```python
from build123d import *

# Parameters (mm, degrees)
F1_DEPTH = 3.175
F2_W     = 3.175
F2_H     = 25.4
F3_DEPTH = 7.62
F2_R     = 1.27
F4_DEPTH = 7.62
F5_R     = 2.15265
F6_DEPTH = 25.4


# Not quite as in the source:
# - a length typed as a fraction of an inch, garbled in the dataset ("3 / 203.2 mm" for 3/8 in), is restored


with BuildPart() as f1:
    # F0 (on Top) → F1 (new body)
    with BuildSketch(Plane.XY):
        Polygon((-25.4, -43.9940905122), (25.4, -43.9940905122), (50.8, 0), (101.6, 0), (127, 43.9940905122), (101.6, 87.9881810245), (50.8, 87.9881810245), (25.4, 131.9822715367), (-25.4, 131.9822715367), (-50.8, 87.9881810245), (-101.6, 87.9881810245), (-127, 43.9940905122), (-101.6, 0), (-50.8, 0), align=None)
    extrude(amount=F1_DEPTH)

    # F2 (on face) → F3 (cut)
    with BuildSketch(Plane.XY.offset(3.175)):
        with Locations((-21.59, 69.3940905122)):
            Rectangle(F2_W, F2_H)
        with Locations((21.59, 69.3940905122)):
            Rectangle(F2_W, F2_H)
        with Locations((21.59, 18.5940905122)):
            Rectangle(F2_W, F2_H)
        with Locations((-21.59, 18.5940905122)):
            Rectangle(F2_W, F2_H)
    extrude(amount=-F3_DEPTH, mode=Mode.SUBTRACT)

    # F2 (on face) → F4 (cut)
    with BuildSketch(Plane.XY.offset(3.175)):
        with Locations((-21.59, 43.9940905122)):
            Circle(F2_R)
        with Locations((21.59, 43.9940905122)):
            Circle(F2_R)
    extrude(amount=-F4_DEPTH, mode=Mode.SUBTRACT)

    # F5 (on face) → F6 (cut)
    with BuildSketch(Plane.XY.offset(3.175)):
        with Locations((97.79, 66.0370998967)):
            Circle(F5_R)
        with Locations((-97.79, 66.0370998967)):
            Circle(F5_R)
    extrude(amount=-F6_DEPTH, mode=Mode.SUBTRACT)


solid = f1.part
```
Check sheet for the modelled part. Datum: model origin and axes. Units: mm. Coordinates: 2 decimals unless noted, no trailing zeros. Loops run counter-clockwise (first coordinate to the right, second up) from the corner with the lowest first, then second, coordinate; pieces in that order, holes last.
1) Gauge pin test, flat ends, axial feed: pin 1 (1 mm diameter, centred on y = 75.5, z = 2, fed in from +X); pin 2 (1.6 mm diameter, centred on x = -85, z = 1, fed in from -Y); pin 3 (1.6 mm diameter, centred on x = -71, z = 1.5, fed in from +Y); pin 4 (2 mm diameter, centred on x = 21.59, y = 43.99, fed in from -Z). Record the tip position at first contact, or that the pin passes through.
2) Sectioned sample at D-D (y = -14). Record the boundary of the cut face in (x, z) (3 decimals).
3) Material ranges on probe 1 along Y at (x, z) = (-21.59, 2.4); probe 2 along X at (y, z) = (10.5, 1.6); probe 3 along Y at (x, z) = (95, 1.7), recorded low to high.
4) Sectioned sample at B-B (z = 0.75). Count the separate pieces of the cut face and the enclosed holes in it, and give its area (3 significant figures).
5) Sectioned sample at C-C (x = -82). Record the boundary of the cut face in (y, z) (3 decimals).
6) Sectioned sample at A-A (y = 72). Record the boundary of the cut face in (x, z) (1 decimal).
Check sheet entries:
1. pin 1: stops at x = 109.1
1. pin 2: stops at y = 0
1. pin 3: stops at y = 87.99
1. pin 4: passes through
2. outline: (-42.717, 0) - (42.717, 0) - (42.717, 3.175) - (-42.717, 3.175) - close
3. probe 1: y = -43.99 to 5.89, 31.29 to 42.72, 45.26 to 56.69, 82.09 to 131.98
3. probe 2: x = -107.66 to -23.18, -20 to 20, 23.18 to 107.66
3. probe 3: y = 0 to 87.99
4. separate pieces: 1
4. enclosed holes: 8
4. area: 26,500 mm2
5. outline: (0, 0) - (87.988, 0) - (87.988, 3.175) - (0, 3.175) - close
6. outline: (-110.8, 0) - (-23.2, 0) - (-23.2, 3.2) - (-110.8, 3.2) - close; (-20, 0) - (20, 0) - (20, 3.2) - (-20, 3.2) - close; (23.2, 0) - (110.8, 0) - (110.8, 3.2) - (23.2, 3.2) - close
